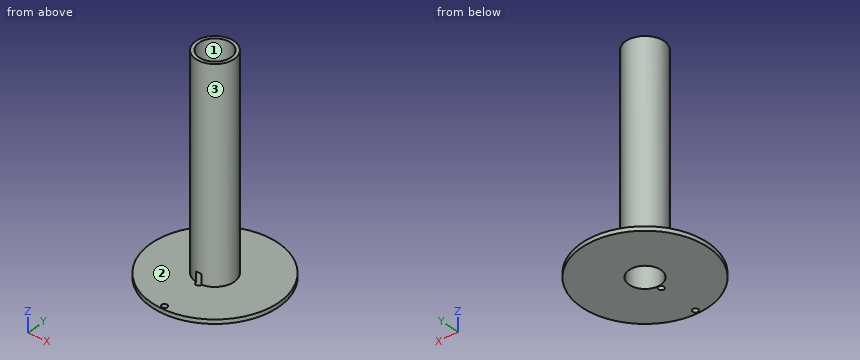
from build123d import *

# Parameters (mm, degrees)
F0_R          = 19.05
F0_R_2        = 5.75
F0_R_3        = 4.75
F1_DEPTH      = 1.25
F2_DEPTH      = 63.5
F3_R          = 0.8507078104
F4_DEPTH      = 25.4
F4_DEPTH_BACK = 3.0226


with BuildPart() as f1:
    # F0 (on Top) → F1 (new body)
    with BuildSketch(Plane.XY):
        Circle(F0_R)
        Circle(F0_R_2, mode=Mode.SUBTRACT)
        Circle(F0_R_2)
        Circle(F0_R_3, mode=Mode.SUBTRACT)
    extrude(amount=F1_DEPTH)

    # F0 (on Top) → F2 (join)
    with BuildSketch(Plane.XY):
        Circle(F0_R_2)
        Circle(F0_R_3, mode=Mode.SUBTRACT)
    extrude(amount=F2_DEPTH)

    # F3 (on face) → F4 (cut, two sides)
    with BuildSketch(Plane.XY.offset(1.25)) as f4_sk:
        with Locations((0, -5.75)):
            Circle(F3_R)
        with Locations((0, -17.8138911724)):
            Circle(F3_R)
    extrude(amount=-F4_DEPTH, mode=Mode.SUBTRACT)
    extrude(f4_sk.sketch, amount=F4_DEPTH_BACK, mode=Mode.SUBTRACT)


solid = f1.part
Geometry: final body of the model. Coordinates: model frame, mm. Face numbers are marked on the shaded views. Round coordinates to 2 decimals unless told otherwise and drop trailing zeros. Loops run counter-clockwise (first coordinate to the right, second up) from the corner with the lowest first, then second, coordinate; pieces in that order, holes last.
Q1. Section A-A on y = 0. Return loops of the section in (x, z), plus the area to 3 significant figures.
Q2. Pull-direction query (X, two-part tool) for the marked faces 1, 2 and 3; classes: released by +X, released by -X, zero draft, split by the parting line, or undercut.
Q3. Section D-D on y = 4. Return loops of the section in (x, z), plus the area to 3 significant figures.
Q4. Section B-B on x = 0. Return loops of the section in (y, z).
Q5. Section C-C on z = 37.5. Return loops of the section in (x, y).
Q6. Pin query (flat end, axial travel): P1, Ø1.4, axis at x = 0, y = -17.81, coming from the -Z side; P2, Ø3, axis at x = 4.5, z = 57, coming from the -Y side; P3, Ø1, axis at y = -1, z = 52.5, coming from the -X side; P4, Ø1, axis at x = -10.5, y = 0.5, coming from the +Z side. Return the tip coordinate at first contact, or that it passes through.
Q7. Material intervals for L1, parallel to Y at x = 0, z = 42; L2, parallel to Z at x = 15, y = -2.5; L3, parallel to X at y = -1, z = 5.5, sorted ascending.
Evaluation:
1. outline: (-19.05, 0) - (-4.75, 0) - (-4.75, 63.5) - (-5.75, 63.5) - (-5.75, 1.25) - (-19.05, 1.25) - close; (4.75, 0) - (19.05, 0) - (19.05, 1.25) - (5.75, 1.25) - (5.75, 63.5) - (4.75, 63.5) - close
1. area: 160 mm2
2. face 1: undercut
2. face 2: zero draft
2. face 3: split by the parting line
3. outline: (-18.63, 0) - (-2.56, 0) - (-2.56, 63.5) - (-4.13, 63.5) - (-4.13, 1.25) - (-18.63, 1.25) - close; (2.56, 0) - (18.63, 0) - (18.63, 1.25) - (4.13, 1.25) - (4.13, 63.5) - (2.56, 63.5) - close
3. area: 235 mm2
4. outline: (-19.05, 0) - (-18.66, 0) - (-18.66, 1.25) - (-19.05, 1.25) - close; (-16.96, 0) - (-6.6, 0) - (-6.6, 1.25) - (-16.96, 1.25) - close; (-5.75, 4.27) - (-4.9, 4.27) - (-4.9, 0) - (-4.75, 0) - (-4.75, 63.5) - (-5.75, 63.5) - close; (4.75, 0) - (19.05, 0) - (19.05, 1.25) - (5.75, 1.25) - (5.75, 63.5) - (4.75, 63.5) - close
5. outline: circle Ø11.5 at (0, 0); hole circle Ø9.5 at (0, 0)
6. P1: passes through
6. P2: stops at y = -4.91
6. P3: stops at x = -5.73
6. P4: stops at z = 1.25
7. L1: y = -5.75 to -4.75, 4.75 to 5.75
7. L2: z = 0 to 1.25
7. L3: x = -5.66 to -4.64, 4.64 to 5.66
